from build123d import *

# Parameters (mm, degrees)
ESQUISSE1_R               = 1.5
EXTRUSION1_DEPTH          = 5
ESQUISSE2_R               = 2.9
ENL_V_MAT_EXTRU_1_DEPTH   = 29.176940927
TROU_TARAUD_M3X0_51_D     = 2.5
TROU_TARAUD_M3X0_51_DEPTH = 9.1
TROU_TARAUD_M3X0_51_TIP   = 0.751075774


with BuildPart() as part:
    # Esquisse1 → Extrusion1 (new body)
    with BuildSketch(Plane.XY):
        with BuildLine():
            Line((0.799950986, 7.959904423), (-19.5, 10))
            Line((-19.5, 10), (-19.5, -20))
            Line((-19.5, -20), (3.888568512, -6.991354299))
            ThreePointArc((3.888568512, -6.991354299), (7.834576447, 1.618459728), (0.799950986, 7.959904423))
        make_face()
        Circle(ESQUISSE1_R, mode=Mode.SUBTRACT)
    extrude(amount=-EXTRUSION1_DEPTH)

    # Esquisse2 → Enlèv. mat.-Extru.1 (cut, through all)
    with BuildSketch(Plane(origin=(0, 0, -3.7), x_dir=(-1, 0, 0), z_dir=(0, 0, -1))):
        Circle(ESQUISSE2_R)
    extrude(amount=-ENL_V_MAT_EXTRU_1_DEPTH, mode=Mode.SUBTRACT)

    # Trou taraudé M3x0.51
    with Locations(Plane.ZY.offset(19.5)):
        with Locations((-2.5, 6), (-2.5, -16)):
            Hole(TROU_TARAUD_M3X0_51_D / 2, depth=TROU_TARAUD_M3X0_51_DEPTH)
            with Locations((0, 0, -(TROU_TARAUD_M3X0_51_DEPTH + TROU_TARAUD_M3X0_51_TIP / 2))):  # 118° drill point
                Cone(0, TROU_TARAUD_M3X0_51_D / 2, TROU_TARAUD_M3X0_51_TIP, mode=Mode.SUBTRACT)


solid = part.part
Design review of the part built by this model. Coordinates are the model's own, in mm. A direction names the side the tool comes from. Round coordinates to 2 decimals unless told otherwise and drop trailing zeros. Write each loop counter-clockwise with the first axis right and the second up, starting at its lowest first coordinate (ties: lowest second). Pieces come first, ordered by that corner, then holes. Notation, with made-up numbers: (1, 89.5) -> (30, 89.5) arc R24 cw to (30, 119.5) -> close; hole circle Ø4 at (37, 78.5). An arc over 180 degrees is marked (long way). One line per question, with ' | ' between items.
(1) Wall thickness on line 1 (Z direction, x = -15.25, y = 6); line 2 (X direction, y = 1.25, z = -2.6); line 3 (Y direction, x = -12, z = -2.1): over which ranges is each line inside the solid? List them lowest first. Write a range as [from, to].
Result sheet:
line 1: [-5, -3.75], [-1.25, 0] | line 2: [-19.5, -2.62], [2.62, 7.9] | line 3: [-14.82, 4.82], [7.18, 9.25]
(2) Take a section at D-D, the plane y = -16. State the section outline as (x, z) points.
Result sheet:
outline: (-19.5, -5) -> (-12.31, -5) -> (-12.31, -3.75) -> (-19.5, -3.75) -> close; (-19.5, -1.25) -> (-12.31, -1.25) -> (-12.31, 0) -> (-19.5, 0) -> close
(3) Take a section at A-A, the plane y = 0. State the section outline as (x, z) points, and give its area (3 significant figures).
Result sheet:
outline: (-19.5, -5) -> (-1.5, -5) -> (-1.5, -3.7) -> (-2.9, -3.7) -> (-2.9, 0) -> (-19.5, 0) -> close; (1.5, -5) -> (8, -5) -> (8, 0) -> (2.9, 0) -> (2.9, -3.7) -> (1.5, -3.7) -> close | area: 112 mm2
(4) Take a section at C-C, the plane x = -13.5. State the section outline as (y, z) points.
Result sheet:
outline: (-16.66, -5) -> (9.4, -5) -> (9.4, 0) -> (-16.66, 0) -> (-16.66, -1.44) arc R1.25 cw (long way) to (-16.66, -3.56) -> close; hole circle Ø2.5 at (6, -2.5)
(5) Draft analysis for pull direction X (two halves, no side actions). For faces 1 (the conical face through (-9.78, 6.15, -2.66)), 2 (the cylindrical face through (-1.5, 0.07, -4.34)), 3 (the cylindrical face through (-14.886, 4.891, -3.077)), 4 (the flat face through (-9.208, 8.966, -2.465)), state which applies: released by +X, released by -X, zero draft, split by the parting line, or undercut.
Result sheet:
face 1: released by -X | face 2: undercut | face 3: zero draft | face 4: released by +X
(6) Insertion check: P1, Ø4.5, axis at x = 0, y = 0, coming from the -Z side; P2, Ø2, axis at x = 5, z = -4.5, coming from the -Y side; P3, Ø3, axis at y = 6, z = -2.5, coming from the +X side. Each pin has a flat end and moves straight along its axis. Give the tip position at first contact, or say it passes through.
Result sheet:
P1: z = -5 | P2: y = -6.93 | P3: x = 6.61
(7) Take a section at B-B, the plane x = 0. State the section outline as (y, z) points.
Result sheet:
outline: (-9.15, -5) -> (-1.5, -5) -> (-1.5, -3.7) -> (-2.9, -3.7) -> (-2.9, 0) -> (-9.15, 0) -> close; (1.5, -5) -> (8.04, -5) -> (8.04, 0) -> (2.9, 0) -> (2.9, -3.7) -> (1.5, -3.7) -> close
(8) Machinability: for faces 5 (the flat face through (-9, -1, 0)), 6 (the cylindrical face through (2.9, 0.1, -1.9)), 7 (the cylindrical face through (-15.9, -14.76, -2.34)), which of the approach directions +Z, -Z, +X, -X, +Y, -Y give a long, thin tool a straight path to every point of the face, cutting with its end or side? Answer none if there is none.
Result sheet:
face 5: +Z, +X, -X, +Y, -Y | face 6: +Z | face 7: -X
